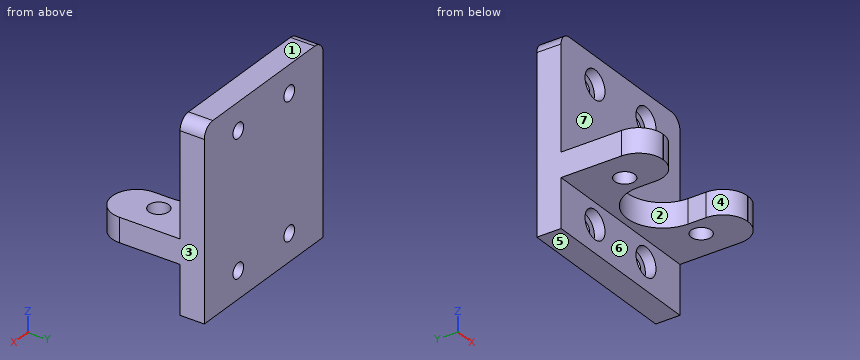
from build123d import *

# Parameters (mm, degrees)
F0_W      = 28
F0_H      = 31
F1_DEPTH  = 4
F3_D      = 2.5
F2_W      = 28
F2_H      = 4
F4_DEPTH  = 14
F6_DEPTH  = 25
F7_D      = 3.3
F8_R      = 4
F9_R      = 2
F2_R      = 2.35
F10_DEPTH = 1.75


with BuildPart() as f1:
    # F0 (on Front) → F1 (new body)
    with BuildSketch(Plane.XZ):
        with Locations((14, 15.5)):
            Rectangle(F0_W, F0_H)
    extrude(amount=F1_DEPTH)

    # F3 (through all)
    with Locations(Plane.XZ.offset(4)):
        with Locations((8, 26.5), (20, 26.5), (20, 4.5), (8, 4.5)):
            Hole(F3_D / 2)

    # F2 (on face) → F4 (join)
    with BuildSketch(Plane.XZ.offset(4)):
        with Locations((14, 10)):
            Rectangle(F2_W, F2_H)
    extrude(amount=F4_DEPTH)

    # F5 (on face) → F6 (cut)
    with BuildSketch(Plane(origin=(0, 0, 8), x_dir=(1, 0, 0), z_dir=(0, 0, -1))):
        with BuildLine():
            ThreePointArc((8.1, 11), (14, 16.9), (19.9, 11))
            Line((19.9, 11), (19.9, 18))
            Line((19.9, 18), (8.1, 18))
            Line((8.1, 18), (8.1, 11))
        make_face()
        with BuildLine():
            ThreePointArc((8.1, 11), (14, 5.1), (19.9, 11))
            ThreePointArc((19.9, 11), (14, 16.9), (8.1, 11))
        make_face()
    extrude(amount=-F6_DEPTH, mode=Mode.SUBTRACT)

    # F7 (through all)
    with Locations(Plane(origin=(0, 0, 8), x_dir=(1, 0, 0), z_dir=(0, 0, -1))):
        with Locations((5, 11), (23, 11)):
            Hole(F7_D / 2)

    # F8
    f8_edges = [f1.edges().sort_by_distance(p)[0] for p in [
        (28, -18, 10),
        (19.9, -18, 10),
        (8.1, -18, 10),
        (0, -18, 10),
    ]]
    fillet(f8_edges, radius=F8_R)

    # F9
    f9_edges = [f1.edges().sort_by_distance(p)[0] for p in [
        (28, -2, 31),
        (0, -2, 31),
    ]]
    fillet(f9_edges, radius=F9_R)

    # F2 (on face) → F10 (cut)
    with BuildSketch(Plane.XZ.offset(4)):
        with Locations((8, 26.5)):
            Circle(F2_R)
        with Locations((20, 26.5)):
            Circle(F2_R)
        with Locations((20, 4.5)):
            Circle(F2_R)
        with Locations((8, 4.5)):
            Circle(F2_R)
    extrude(amount=-F10_DEPTH, mode=Mode.SUBTRACT)


solid = f1.part
Model file for the job. Use its own axes, mm. Face numbers are marked on the shaded views. A direction names the side the tool comes from. Round coordinates to 2 decimals unless told otherwise and drop trailing zeros. Order: outer loops, then holes, each group sorted by start corner. A loop starts at its lowest first (then second) coordinate and runs counter-clockwise, first axis right, second up.
(1) Pin check, flat tips, straight feed: pin 1 (4 mm diameter, centred on x = 23, y = -11, fed in from -Z); pin 2 (1 mm diameter, centred on x = 3.5, z = 4.5, fed in from -Y); pin 3 (1.4 mm diameter, centred on x = 8.5, z = 27, fed in from -Y); pin 4 (3 mm diameter, centred on x = 5, y = -11, fed in from +Z). Stop position of each tip, or through.
(2) Band-saw the part on A-A (y = -13.25). List the corners of the cut face in (x, z), then the cut area to 3 significant figures.
(3) Band-saw the part on C-C (x = 5). List the corners of the cut face in (y, z), then the cut area to 3 significant figures.
(4) Band-saw the part on D-D (y = -10). List the corners of the cut face in (x, z), then the cut area to 3 significant figures.
(5) 3-axis set-ups, long thin cutter, end or side, ignore diameter. For the marked faces 4, 5, 6 and 7: which of +Z, -Z, +X, -X, +Y, -Y reach the whole face in a straight line?
(6) Drill centre lines: line 1 (X direction, y = -11, z = 10.15); line 2 (Z direction, x = 8, y = -0.65); line 3 (Z direction, x = 20, y = -3.25). Where is each one in solid material? Low to high.
(7) Band-saw the part on B-B (z = 4.5). List the corners of the cut face in (x, y), then the cut area to 3 significant figures.
(8) Pull direction X, two halves, no side cores. Call the marked faces 1, 2 and 3: released by +X, released by -X, zero draft, split by the parting line, or undercut.
Verdict:
1. pin 1: stops at z = 8
1. pin 2: stops at y = -4
1. pin 3: stops at y = -2.25
1. pin 4: passes through
2. outline: (0, 8) - (8.1, 8) - (8.1, 12) - (0, 12) - close; (19.9, 8) - (28, 8) - (28, 12) - (19.9, 12) - close
2. area: 64.8 mm2
3. outline: (-17.9, 8) - (-12.65, 8) - (-12.65, 12) - (-17.9, 12) - close; (-9.35, 8) - (-4, 8) - (-4, 0) - (0, 0) - (0, 31) - (-4, 31) - (-4, 12) - (-9.35, 12) - close
3. area: 166 mm2
4. outline: (0, 8) - (3.69, 8) - (3.69, 12) - (0, 12) - close; (6.31, 8) - (8.19, 8) - (8.19, 12) - (6.31, 12) - close; (19.81, 8) - (21.69, 8) - (21.69, 12) - (19.81, 12) - close; (24.31, 8) - (28, 8) - (28, 12) - (24.31, 12) - close
4. area: 44.5 mm2
5. face 4: +Z, -Z, -Y
5. face 5: -Z, +X, -X, +Y, -Y
5. face 6: -Z, +X, -X, -Y
5. face 7: +Z, +X, -X, -Y
6. line 1: x = 0 to 3.35, 6.65 to 8.1, 19.9 to 21.35, 24.65 to 28
6. line 2: z = 0 to 3.25, 5.75 to 25.25, 27.75 to 31
6. line 3: z = 0 to 2.15, 6.85 to 24.15, 28.85 to 31
7. outline: (0, -4) - (5.65, -4) - (5.65, -2.25) - (6.75, -2.25) - (6.75, 0) - (0, 0) - close; (9.25, -2.25) - (10.35, -2.25) - (10.35, -4) - (17.65, -4) - (17.65, -2.25) - (18.75, -2.25) - (18.75, 0) - (9.25, 0) - close; (21.25, -2.25) - (22.35, -2.25) - (22.35, -4) - (28, -4) - (28, 0) - (21.25, 0) - close
7. area: 84.3 mm2
8. face 1: zero draft
8. face 2: undercut
8. face 3: released by +X
